from build123d import *

# Parameters (mm, degrees)
F0_W     = 178.8466324
F0_H     = 155.575
F0_R     = 2.15265
F1_DEPTH = 3.175
F2_R     = 3.96875
F4_DEPTH = 3.175
F5_R     = 0.762
F6_SIZE  = 9.525
F7_R     = 1.7272
F8_DEPTH = 3.175


with BuildPart() as f1:
    # F0 (on Top) → F1 (new body)
    with BuildSketch(Plane.XY):
        with Locations((89.4233162, -77.7875)):
            Rectangle(F0_W, F0_H)
        with Locations((20.8903824, -151.60625)):
            Circle(F0_R, mode=Mode.SUBTRACT)
        with Locations((35.1778824, -151.60625)):
            Circle(F0_R, mode=Mode.SUBTRACT)
        with Locations((160.5903824, -151.60625)):
            Circle(F0_R, mode=Mode.SUBTRACT)
        with Locations((174.8778824, -151.60625)):
            Circle(F0_R, mode=Mode.SUBTRACT)
        with Locations((20.8903824, -3.96875)):
            Circle(F0_R, mode=Mode.SUBTRACT)
        with Locations((35.1778824, -3.96875)):
            Circle(F0_R, mode=Mode.SUBTRACT)
        with Locations((160.5903824, -3.96875)):
            Circle(F0_R, mode=Mode.SUBTRACT)
        with Locations((174.8778824, -3.96875)):
            Circle(F0_R, mode=Mode.SUBTRACT)
    extrude(amount=F1_DEPTH)

    # F2
    f2_edges = [f1.edges().sort_by_distance(p)[0] for p in [
        (178.846632, 0, 1.5875),
        (178.846632, -155.575, 1.5875),
    ]]
    fillet(f2_edges, radius=F2_R)

    # F3 (on face) → F4 (cut, through all)
    with BuildSketch(Plane.XY.offset(3.175)):
        with BuildLine():
            Line((0, -17.8102557702), (0, -137.7647442298))
            ThreePointArc((0, -137.7647442298), (15.9905975048, -130.293948325), (3.175, -118.1583617876))
            Line((3.175, -118.1583617876), (3.175, -37.4166382124))
            ThreePointArc((3.175, -37.4166382124), (15.9905975048, -25.281051675), (0, -17.8102557702))
        make_face()
    extrude(amount=-F4_DEPTH, mode=Mode.SUBTRACT)

    # F5
    f5_edges = [f1.edges().sort_by_distance(p)[0] for p in [
        (0, -17.810256, 1.5875),
        (0, -137.764744, 1.5875),
        (3.175, -37.416638, 1.5875),
        (3.175, -118.158362, 1.5875),
    ]]
    fillet(f5_edges, radius=F5_R)

    # F6
    f6_edges = [f1.edges().sort_by_distance(p)[0] for p in [
        (0, 0, 1.5875),
        (0, -155.575, 1.5875),
    ]]
    chamfer(f6_edges, length=F6_SIZE)

    # F7 (on face) → F8 (cut, through all)
    with BuildSketch(Plane.XY.offset(3.175)):
        with Locations((92.2014412, -4.7625)):
            Circle(F7_R)
        with Locations((14.2875, -4.7625)):
            Circle(F7_R)
        with Locations((14.2875, -150.8125)):
            Circle(F7_R)
        with Locations((92.2014412, -150.8125)):
            Circle(F7_R)
    extrude(amount=-F8_DEPTH, mode=Mode.SUBTRACT)


solid = f1.part
Work out the finished part from the listing and answer in its coordinate system (mm). Give positions to 0.01 mm unless a question says otherwise; leave off trailing zeros. Loops run counter-clockwise (first coordinate to the right, second up) from the corner with the lowest first, then second, coordinate; pieces in that order, holes last. Notation, with made-up numbers: (80, 3.5) -> (91, 3.5) arc R17 ccw to (91, 32.5) -> close; hole circle Ø9 at (-24, -25.5). An arc over 180 degrees is marked (long way). Use a Markdown table: item, result. Add a question column.
1. Find the intervals of material crossed by probe 1 along X at (y, z) = (-108.5, 2.3) (3 decimals); probe 2 along X at (y, z) = (-133, 1.3), in increasing order.
2. Section A-A on z = 1.65 is taken. State how many separate pieces and enclosed holes the cut face has, and give its area (3 significant figures).
3. Section C-C on y = -26.5 is taken. Determine the outline of the cut face in (x, z) (3 decimals), and give its area (3 significant figures).
4. Section B-B on y = -81 is taken. Determine the outline of the cut face in (x, z) (3 decimals).
5. Flat-ended cylindrical pins translate along their axes: pin 1 Ø4 at (x, y) = (20.89, -151.61) entering from +Z; pin 2 Ø1.5 at (x, y) = (89, -27.5) entering from -Z. Find the tip coordinate at first contact, or state that the pin passes through.
6. Determine the mould class of faces 1 (the flat face through (88, -77, 0)), 2 (the cylindrical face through (162.58, -152.43, 1.57)), 3 (the cylindrical face through (177.65, -1.13, 1.61)), 4 (the cylindrical face through (177.653, -154.443, 1.61)) for opening direction Y: released by +Y, released by -Y, zero draft, split by the parting line, or undercut.
Results below:
| question | item | result |
|---|---|---|
| 1 | probe 1 | x = 3.175 to 178.847 |
| 1 | probe 2 | x = 15.17 to 178.85 |
| 2 | separate pieces | 1 |
| 2 | enclosed holes | 12 |
| 2 | area | 26,700 mm^2 |
| 3 | outline | (16.117, 0) -> (178.847, 0) -> (178.847, 3.175) -> (16.117, 3.175) -> close |
| 3 | area | 517 mm^2 |
| 4 | outline | (3.175, 0) -> (178.847, 0) -> (178.847, 3.175) -> (3.175, 3.175) -> close |
| 5 | pin 1 | passes through |
| 5 | pin 2 | stops at z = 0 |
| 6 | face 1 | zero draft |
| 6 | face 2 | undercut |
| 6 | face 3 | released by +Y |
| 6 | face 4 | released by -Y |
